Autodesk Inventor part; units mm, degrees
ref_plane "YZ Plane" through (0, 0, 0) normal (1, 0, 0) x (0, 1, 0)
ref_plane "XZ Plane" through (0, 0, 0) normal (0, 1, 0) x (-1, 0, 0)
ref_plane "XY Plane" through (0, 0, 0) normal (0, 0, 1) x (1, 0, 0)
ref_plane "Arbeitsebene3" through (0, 0, 0) normal (0, 0, 1) x (1, 0, 0)
sketch "Skizze1" plane through (0, 0, 0) normal (0, 0, 1) x (1, 0, 0)
  circle A0 centre (871.1765, 73.7926) radius 2.6 construction
  circle A1 centre (881.1765, 21.442) radius 2.6 construction
  circle A2 centre (28.8235, 21.442) radius 2.6 construction
  circle A3 centre (38.8235, 73.7926) radius 2.6 construction
  line L0 (910, 0) -> (0, 0) construction
  line L1 (910, 0) -> (910, 139) construction
  line L2 (0, 139) -> (910, 139) construction
  line L3 (0, 0) -> (0, 139) construction
  circle A4 centre (-21.0024, 109.9626) radius 6 construction
  line L4 (0, 134.7877) -> (0, 139)
  line L5 (0, 141.9626) -> (-2.1715, 141.9626)
  line L6 (12.5314, 139) -> (0, 139)
  line L7 (0, 141.9626) -> (12.5314, 141.9626)
  line L8 (12.5314, 141.9626) -> (12.5314, 139)
  line L9 (-12.3384, 111.9626) -> (-12.3384, 119.1463)
  line L10 (-12.3384, 119.1463) -> (0, 134.7877)
  line L11 (-21.0024, 109.9626) -> (-21.0024, 111.9626) construction
  arc A5 (-14.8524, 111.9626) -> (-27.1524, 111.9626) centre (-21.0024, 111.9626) ccw
  line L12 (-30.2709, 111.9626) -> (-30.2709, 113.0226)
  line L13 (-30.2709, 113.0226) -> (-2.1715, 141.9626)
  arc A6 (-27.0706, 110.9626) -> (-27.1524, 111.9626) centre (-21.0024, 111.9626) ccw construction
  line L14 (-27.1524, 111.9626) -> (-30.2709, 111.9626)
  line L15 (-14.8524, 111.9626) -> (-12.3384, 111.9626)
extrude "Extrusion1" add sketch "Skizze1" against normal blind 10
sketch "Skizze2" plane through (0, 0, -10) normal (0, 0, -1) x (-1, 0, 0)
  line L0 (2.1715, 141.9626) -> (-12.5314, 141.9626) construction
  line L1 (-12.5314, 141.9626) -> (-12.5314, 139) construction
  line L2 (-12.5314, 139) -> (0, 139) construction
  line L3 (0, 139) -> (0, 134.7877) construction
  line L4 (0, 134.7877) -> (12.3384, 119.1463) construction
  line L5 (12.3384, 119.1463) -> (12.3384, 111.9626) construction
  line L6 (12.3384, 111.9626) -> (14.8524, 111.9626) construction
  arc A0 (27.1524, 111.9626) -> (14.8524, 111.9626) centre (21.0024, 111.9626) ccw construction
  line L7 (27.1524, 111.9626) -> (30.2709, 111.9626) construction
  line L8 (30.2709, 111.9626) -> (30.2709, 113.0226) construction
  line L9 (30.2709, 113.0226) -> (2.1715, 141.9626) construction
  line L10 (2.6888, 135.6545) -> (14.0699, 121.2268)
  line L11 (4.2009, 136.8473) -> (2.6888, 135.6545)
  line L12 (4.2009, 136.8473) -> (19.3387, 121.2268)
  line L13 (19.3387, 121.2268) -> (14.0699, 121.2268)
  point P0 (0, 0)
extrude "Extrusion2" cut sketch "Skizze2" against normal through all
properties part number "Lin_gage"
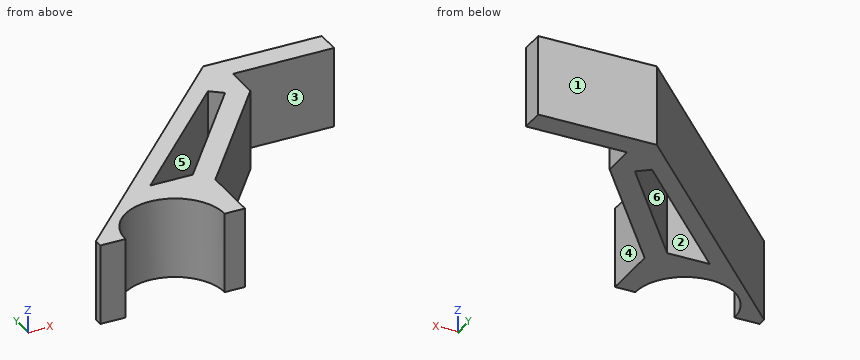
Geometry: final body of the model. Coordinates: model frame, mm. Face numbers are marked on the shaded views. A direction names the side the tool comes from. Give positions to 0.01 mm unless a question says otherwise; leave off trailing zeros. Write each loop counter-clockwise with the first axis right and the second up, starting at its lowest first coordinate (ties: lowest second). Pieces come first, ordered by that corner, then holes. Notation, with made-up numbers: M -39.75,-39.75 L -7.75,-39.75 A24 cw -7.75,-23.75 Z; hole C 56,88.25 d3. An arc over 180 degrees is marked long. Answer in a Markdown table with one row per item. Add a question column.
(1) Reachability of the marked faces 1 and 2 from +Z, -Z, +X, -X, +Y, -Y: full face, straight path, thin tool, end or side. Return the list, or none.
(2) First-contact query: pin 1 (3 mm diameter, centred on x = -20, y = 122, fed in from +Z); pin 2 (1.5 mm diameter, centred on y = 128.5, z = -1, fed in from +X); pin 3 (4 mm diameter, centred on y = 136.5, z = -5, fed in from -X); pin 4 (3 mm diameter, centred on y = 126, z = -9, fed in from +X). Flat tips, straight axial feed; report the tip coordinate or a pass-through.
(3) Section A-A on z = -2.5. Return loops of the section in (x, y).
(4) Mould query, pull axis Y, two halves, no side actions, for the marked faces 3, 4, 5 and 6. Classes: +Y half, -Y half, draft (parallel to the pull), parting line (faces both ways), or undercut.
(5) Section D-D on x = 7.5. Return loops of the section in (y, z), and give its area (3 significant figures).
(6) Section B-B on x = -7. Return loops of the section in (y, z), and give its area (3 significant figures).
(7) Ray query, line 1 (Y direction, x = -16, z = -7); line 2 (X direction, y = 116, z = -5); line 3 (X direction, y = 113, z = -6.75). Return the intervals inside material, ascending.
(8) Section C-C on y = 128. Return loops of the section in (x, z).
Result set:
| question | item | result |
|---|---|---|
| 1 | face 1 | +Z, -Z, +X, -X, +Y |
| 1 | face 2 | +Z, -Z |
| 2 | pin 1 | stops at z = 0 |
| 2 | pin 2 | stops at x = -4.37 |
| 2 | pin 3 | stops at x = -9.42 |
| 2 | pin 4 | stops at x = -5.75 |
| 3 | outline | M -30.27,111.96 L -27.15,111.96 A6.15 cw -14.85,111.96 L -12.34,111.96 L -12.34,119.15 L 0,134.79 L 0,139 L 12.53,139 L 12.53,141.96 L -2.17,141.96 L -30.27,113.02 Z; hole M -19.34,121.23 L -14.07,121.23 L -2.69,135.65 L -4.2,136.85 Z |
| 4 | face 3 | -Y half |
| 4 | face 4 | draft |
| 4 | face 5 | undercut |
| 4 | face 6 | undercut |
| 5 | outline | M 139,-10 L 141.96,-10 L 141.96,0 L 139,0 Z |
| 5 | area | 29.6 mm^2 |
| 6 | outline | M 125.91,-10 L 130.19,-10 L 130.19,0 L 125.91,0 Z; M 133.96,-10 L 136.99,-10 L 136.99,0 L 133.96,0 Z |
| 6 | area | 73.1 mm^2 |
| 7 | line 1 | y = 115.54 to 121.23, 124.67 to 127.72 |
| 7 | line 2 | x = -27.38 to -25.64, -16.36 to -12.34 |
| 7 | line 3 | x = -30.27 to -27.06, -14.94 to -12.34 |
| 8 | outline | M -15.73,-10 L -12.77,-10 L -12.77,0 L -15.73,0 Z; M -8.73,-10 L -5.35,-10 L -5.35,0 L -8.73,0 Z |
